Verification items for the finished model (mm, model axes). Coordinates: 2 decimals unless noted, no trailing zeros. Order: outer loops, then holes, each group sorted by start corner. A loop starts at its lowest first (then second) coordinate and runs counter-clockwise, first axis right, second up. Notation, with made-up numbers: (47.5, 12) -> (92.5, 12) arc R21 ccw to (92.5, 27) -> close; hole circle Ø8 at (-9.5, -20). An arc over 180 degrees is marked (long way). Answer as CSV lines item,"result".
```python
from build123d import *

# Parameters (mm, degrees)
SKETCH1_W               = 156
SKETCH1_H               = 210
BOSS_EXTRUDE1_DEPTH     = 10
SKETCH2_W               = 10
SKETCH2_H               = 10
BOSS_EXTRUDE2_DEPTH     = 10
SKETCH3_R               = 1.75
CUT_EXTRUDE1_DEPTH      = 11
CUT_EXTRUDE1_DEPTH_BACK = 11
CUT_EXTRUDE2_START      = 10
SKETCH4_R               = 3.5
SKETCH4_R_2             = 2.952582507
SKETCH4_R_3             = 2.953821107
CUT_EXTRUDE2_DEPTH      = 3
SKETCH5_R               = 1.75
SKETCH5_W               = 41
SKETCH5_H               = 98
CUT_EXTRUDE3_DEPTH      = 11
CUT_EXTRUDE3_DEPTH_BACK = 11
CUT_EXTRUDE4_START      = 10
SKETCH6_R               = 3.5
CUT_EXTRUDE4_DEPTH      = 3


with BuildPart() as part:
    # Sketch1 → Boss-Extrude1 (new body)
    with BuildSketch(Plane.XY):
        Rectangle(SKETCH1_W, SKETCH1_H)
    extrude(amount=BOSS_EXTRUDE1_DEPTH)

    # Sketch2 → Boss-Extrude2 (add)
    with BuildSketch(Plane.XY):
        with Locations((-73, 0)):
            Rectangle(SKETCH2_W, SKETCH2_H)
        with Locations((73, 0)):
            Rectangle(SKETCH2_W, SKETCH2_H)
    extrude(amount=-BOSS_EXTRUDE2_DEPTH)

    # Sketch3 → Cut-Extrude1 (cut, two sides)
    with BuildSketch(Plane.XY) as cut_extrude1_sk:
        with Locations((-73, 95)):
            Circle(SKETCH3_R)
        with Locations((73, 95)):
            Circle(SKETCH3_R)
        with Locations((73, -95)):
            Circle(SKETCH3_R)
        with Locations((-73, -95)):
            Circle(SKETCH3_R)
    extrude(amount=CUT_EXTRUDE1_DEPTH, mode=Mode.SUBTRACT)
    extrude(cut_extrude1_sk.sketch, amount=-CUT_EXTRUDE1_DEPTH_BACK, mode=Mode.SUBTRACT)

    # Sketch4 → Cut-Extrude2 (cut)
    with BuildSketch(Plane.XY.offset(CUT_EXTRUDE2_START)):
        with Locations((-73, 95)):
            Circle(SKETCH4_R)
        with Locations((73, 95)):
            Circle(SKETCH4_R)
        with Locations((73, -95)):
            Circle(SKETCH4_R_2)
        with Locations((-73, -95)):
            Circle(SKETCH4_R_3)
    extrude(amount=-CUT_EXTRUDE2_DEPTH, mode=Mode.SUBTRACT)

    # Sketch5 → Cut-Extrude3 (cut, two sides)
    with BuildSketch(Plane.XY) as cut_extrude3_sk:
        with Locations((-27.5, 72.5)):
            Circle(SKETCH5_R)
        with Locations((27.5, 72.5)):
            Circle(SKETCH5_R)
        with Locations((27.5, -20.5)):
            Circle(SKETCH5_R)
        with Locations((-27.5, -20.5)):
            Circle(SKETCH5_R)
        with Locations((-20.25, -29.5)):
            Circle(SKETCH5_R)
        with Locations((20.25, -29.5)):
            Circle(SKETCH5_R)
        with Locations((20.25, -95)):
            Circle(SKETCH5_R)
        with Locations((-20.25, -95)):
            Circle(SKETCH5_R)
        with Locations((0, 26)):
            Rectangle(SKETCH5_W, SKETCH5_H)
        with BuildLine():
            Line((10, -39.5), (10, -85))
            ThreePointArc((10, -85), (0, -95), (-10, -85))
            Line((-10, -85), (-10, -39.5))
            ThreePointArc((-10, -39.5), (0, -29.5), (10, -39.5))
        make_face()
    extrude(amount=CUT_EXTRUDE3_DEPTH, mode=Mode.SUBTRACT)
    extrude(cut_extrude3_sk.sketch, amount=-CUT_EXTRUDE3_DEPTH_BACK, mode=Mode.SUBTRACT)

    # Sketch6 → Cut-Extrude4 (cut)
    with BuildSketch(Plane.XY.offset(CUT_EXTRUDE4_START)):
        with Locations((-20.25, -95)):
            Circle(SKETCH6_R)
        with Locations((20.25, -95)):
            Circle(SKETCH6_R)
        with Locations((20.25, -29.5)):
            Circle(SKETCH6_R)
        with Locations((-20.25, -29.5)):
            Circle(SKETCH6_R)
        with Locations((27.5, -20.5)):
            Circle(SKETCH6_R)
        with Locations((-27.5, -20.5)):
            Circle(SKETCH6_R)
        with Locations((-27.5, 72.5)):
            Circle(SKETCH6_R)
        with Locations((27.5, 72.5)):
            Circle(SKETCH6_R)
    extrude(amount=-CUT_EXTRUDE4_DEPTH, mode=Mode.SUBTRACT)


solid = part.part
```
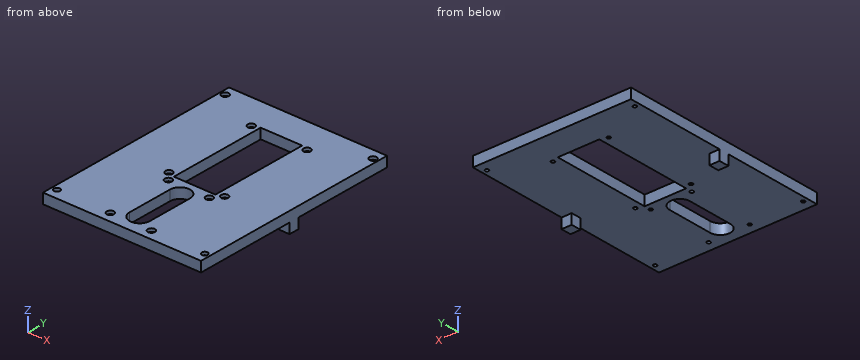
Item 1: Section check A-A, the plane y = -75. Record the boundary of the cut face in (x, z), plus the area to 3 significant figures.
Answer list:
outline,"(-78, 0) -> (-10, 0) -> (-10, 10) -> (-78, 10) -> close; (10, 0) -> (78, 0) -> (78, 10) -> (10, 10) -> close"
area,"1,360 mm2"
Item 2: Depth check by flat-ended pin: pin 1 Ø4.5 at (x, y) = (-27.5, 72.5) entering from +Z; pin 2 Ø4 at (x, y) = (20.25, -95) entering from -Z; pin 3 Ø5 at (x, z) = (74, -5) entering from +Y. Enter the tip coordinate at first touch or a pass-through.
Answer list:
pin 1,"z = 7"
pin 2,"z = 0"
pin 3,"y = 5"
Item 3: Section check C-C, the plane x = -48.5. Record the boundary of the cut face in (y, z).
Answer list:
outline,"(-105, 0) -> (105, 0) -> (105, 10) -> (-105, 10) -> close"
Item 4: Section check B-B, the plane z = -3. Record the boundary of the cut face in (x, y), plus the area to 3 significant figures.
Answer list:
outline,"(-78, -5) -> (-68, -5) -> (-68, 5) -> (-78, 5) -> close; (68, -5) -> (78, -5) -> (78, 5) -> (68, 5) -> close"
area,"200 mm2"
Item 5: Thickness scan on line 1 (Y direction, x = -73, z = 3.25); line 2 (Y direction, x = -20.25, z = 9.15); line 3 (X direction, y = 95, z = 3.25). Record the ranges inside material, lowest first.
Answer list:
line 1,"-105 to -96.75, -93.25 to 93.25, 96.75 to 105"
line 2,"-105 to -98.5, -91.5 to -33, -26 to -23, 75 to 105"
line 3,"-78 to -74.75, -71.25 to 71.25, 74.75 to 78"
